Geometry check sheet. Reference: the model listing, model coordinates, mm. Round coordinates to 2 decimals unless told otherwise and drop trailing zeros. Loops run counter-clockwise (first coordinate to the right, second up) from the corner with the lowest first, then second, coordinate; pieces in that order, holes last. Notation, with made-up numbers: (-2, 78.25) -> (50, 78.25) arc R30 cw to (50, 107.25) -> close; hole circle Ø8 at (5.5, -11.75). An arc over 180 degrees is marked (long way). Use one line per item in the form item = value.
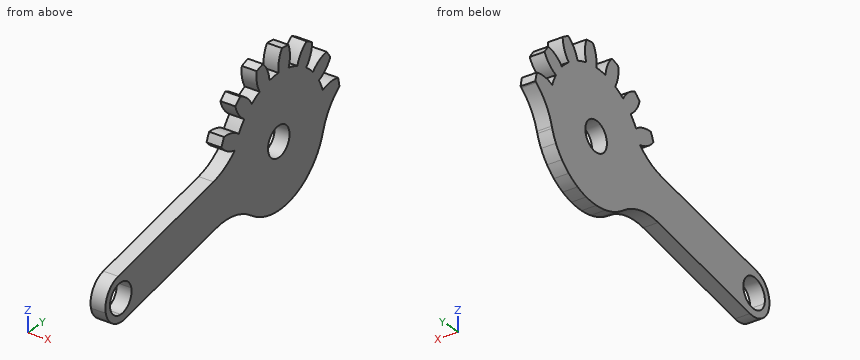
from build123d import *

# Parameters (mm, degrees)
SKETCH1_R           = 1.5
BOSS_EXTRUDE1_DEPTH = 2
SKETCH3_OUTSIDE_W   = 31.914
SKETCH3_OUTSIDE_H   = 31.796
SKETCH3_OUTSIDE_R   = 11.40725
CUT_EXTRUDE1_DEPTH  = 17.630863493
SKETCH4_R           = 2
CUT_EXTRUDE2_DEPTH  = 17.245136509
BOSS_EXTRUDE3_DEPTH = 2
CUT_EXTRUDE3_DEPTH  = 35.211805454
FILLET1_R           = 8


with BuildPart() as part:
    # Sketch1 → Boss-Extrude1 (new body)
    with BuildSketch(Plane(origin=(-1.354941904, 0, 0), x_dir=(0, 0, -1), z_dir=(1, 0, 0))):
        with BuildLine():
            ThreePointArc((-11.66138775, 0.780827758), (-10.210393031, 0.057188521), (-8.592596732, -0.051322118))
            ThreePointArc((-8.592596732, -0.051322118), (-8.545678016, -0.898186953), (-8.415498346, -1.736300708))
            ThreePointArc((-8.415498346, -1.736300708), (-9.975381284, -2.178798893), (-11.24421523, -3.188303642))
            ThreePointArc((-11.24421523, -3.188303642), (-11.115473034, -3.611636122), (-10.97079907, -4.029792056))
            ThreePointArc((-10.97079907, -4.029792056), (-9.350918841, -4.100696673), (-7.828853128, -3.541809038))
            ThreePointArc((-7.828853128, -3.541809038), (-7.441539788, -4.296375), (-6.981723166, -5.009081172))
            ThreePointArc((-6.981723166, -5.009081172), (-8.226766912, -6.047784929), (-8.975301827, -7.486094667))
            ThreePointArc((-8.975301827, -7.486094667), (-8.685505148, -7.820463962), (-8.383259564, -8.143624213))
            ThreePointArc((-8.383259564, -8.143624213), (-6.874585833, -7.549534157), (-5.711429695, -6.419884999))
            ThreePointArc((-5.711429695, -6.419884999), (-5.050691727, -6.951680778), (-4.340744624, -7.415745996))
            ThreePointArc((-4.340744624, -7.415745996), (-5.055669804, -8.871054007), (-5.154477201, -10.489471914))
            ThreePointArc((-5.154477201, -10.489471914), (-4.753734516, -10.677062536), (-4.34617832, -10.849349762))
            ThreePointArc((-4.34617832, -10.849349762), (-3.209574481, -9.692988601), (-2.606448181, -8.187904521))
            ThreePointArc((-2.606448181, -8.187904521), (-1.786533181, -8.404977796), (-0.949211902, -8.540160966))
            ThreePointArc((-0.949211902, -8.540160966), (-1.010401457, -10.160437258), (-0.442396639, -11.679124174))
            ThreePointArc((-0.442396639, -11.679124174), (0, -11.6875), (0.442396639, -11.679124174))
            ThreePointArc((0.442396639, -11.679124174), (1.010401457, -10.160437258), (0.949211902, -8.540160966))
            ThreePointArc((0.949211902, -8.540160966), (1.786533181, -8.404977796), (2.606448181, -8.187904521))
            ThreePointArc((2.606448181, -8.187904521), (3.209574481, -9.692988601), (4.34617832, -10.849349762))
            ThreePointArc((4.34617832, -10.849349762), (4.753734516, -10.677062536), (5.154477201, -10.489471914))
            ThreePointArc((5.154477201, -10.489471914), (5.055669804, -8.871054007), (4.340744624, -7.415745996))
            ThreePointArc((4.340744624, -7.415745996), (5.050691727, -6.951680778), (5.711429695, -6.419884999))
            ThreePointArc((5.711429695, -6.419884999), (6.874585833, -7.549534157), (8.383259564, -8.143624213))
            ThreePointArc((8.383259564, -8.143624213), (8.685505148, -7.820463962), (8.975301827, -7.486094667))
            ThreePointArc((8.975301827, -7.486094667), (8.226766912, -6.047784929), (6.981723166, -5.009081172))
            ThreePointArc((6.981723166, -5.009081172), (7.441539788, -4.296375), (7.828853128, -3.541809038))
            ThreePointArc((7.828853128, -3.541809038), (9.350918841, -4.100696673), (10.97079907, -4.029792056))
            ThreePointArc((10.97079907, -4.029792056), (11.115473034, -3.611636122), (11.24421523, -3.188303642))
            ThreePointArc((11.24421523, -3.188303642), (9.975381284, -2.178798893), (8.415498346, -1.736300708))
            ThreePointArc((8.415498346, -1.736300708), (8.545678016, -0.898186953), (8.592596732, -0.051322118))
            ThreePointArc((8.592596732, -0.051322118), (10.210393031, 0.057188521), (11.66138775, 0.780827758))
            ThreePointArc((11.66138775, 0.780827758), (11.623474652, 1.221676414), (11.568901669, 1.660774047))
            ThreePointArc((11.568901669, 1.660774047), (9.999161608, 2.066921265), (8.394157409, 1.836701922))
            ThreePointArc((8.394157409, 1.836701922), (8.17219088, 2.655305778), (7.8706023, 3.448038862))
            ThreePointArc((7.8706023, 3.448038862), (9.304397507, 4.205185299), (10.335616548, 5.456435359))
            ThreePointArc((10.335616548, 5.456435359), (10.121671907, 5.84375), (9.893219909, 6.222688815))
            ThreePointArc((9.893219909, 6.222688815), (8.29399605, 5.955251959), (6.921390398, 5.092122104))
            ThreePointArc((6.921390398, 5.092122104), (6.385657699, 5.749672018), (5.787709228, 6.351202599))
            ThreePointArc((5.787709228, 6.351202599), (6.789587127, 7.626067336), (7.222723349, 9.188575716))
            ThreePointArc((7.222723349, 9.188575716), (6.869740136, 9.455386122), (6.506910549, 9.708644156))
            ThreePointArc((6.506910549, 9.708644156), (5.154723227, 8.813865487), (4.251852108, 7.467068114))
            ThreePointArc((4.251852108, 7.467068114), (3.49498629, 7.849867731), (2.704068651, 8.156185707))
            ThreePointArc((2.704068651, 8.156185707), (3.100795451, 9.728333051), (2.860955666, 11.331927856))
            ThreePointArc((2.860955666, 11.331927856), (2.429967886, 11.432100084), (1.995497243, 11.515886722))
            ThreePointArc((1.995497243, 11.515886722), (1.124151929, 10.148481601), (0.847129962, 8.55089021))
            ThreePointArc((0.847129962, 8.55089021), (0, 8.59275), (-0.847129962, 8.55089021))
            ThreePointArc((-0.847129962, 8.55089021), (-1.124151929, 10.148481601), (-1.995497243, 11.515886722))
            ThreePointArc((-1.995497243, 11.515886722), (-2.429967886, 11.432100084), (-2.860955666, 11.331927856))
            ThreePointArc((-2.860955666, 11.331927856), (-3.100795451, 9.728333051), (-2.704068651, 8.156185707))
            ThreePointArc((-2.704068651, 8.156185707), (-3.49498629, 7.849867731), (-4.251852108, 7.467068114))
            ThreePointArc((-4.251852108, 7.467068114), (-5.154723227, 8.813865487), (-6.506910549, 9.708644156))
            ThreePointArc((-6.506910549, 9.708644156), (-6.869740136, 9.455386122), (-7.222723349, 9.188575716))
            ThreePointArc((-7.222723349, 9.188575716), (-6.789587127, 7.626067336), (-5.787709228, 6.351202599))
            ThreePointArc((-5.787709228, 6.351202599), (-6.385657699, 5.749672018), (-6.921390398, 5.092122104))
            ThreePointArc((-6.921390398, 5.092122104), (-8.29399605, 5.955251959), (-9.893219909, 6.222688815))
            ThreePointArc((-9.893219909, 6.222688815), (-10.121671907, 5.84375), (-10.335616548, 5.456435359))
            ThreePointArc((-10.335616548, 5.456435359), (-9.304397507, 4.205185299), (-7.8706023, 3.448038862))
            ThreePointArc((-7.8706023, 3.448038862), (-8.17219088, 2.655305778), (-8.394157409, 1.836701922))
            ThreePointArc((-8.394157409, 1.836701922), (-9.999161608, 2.066921265), (-11.568901669, 1.660774047))
            ThreePointArc((-11.568901669, 1.660774047), (-11.623474652, 1.221676414), (-11.66138775, 0.780827758))
        make_face()
        with Locations(Location((0, 0, 0), (0, 0, 180))):
            Circle(SKETCH1_R, mode=Mode.SUBTRACT)
    extrude(amount=-BOSS_EXTRUDE1_DEPTH)

    # Sketch3 outside → Cut-Extrude1 (cut, through all)
    with BuildSketch(Plane(origin=(-1.354941904, 0, 0), x_dir=(0, 0, -1), z_dir=(1, 0, 0))):
        with Locations((0, -0.086)):
            Rectangle(SKETCH3_OUTSIDE_W, SKETCH3_OUTSIDE_H)
        Circle(SKETCH3_OUTSIDE_R, mode=Mode.SUBTRACT)
    extrude(amount=-CUT_EXTRUDE1_DEPTH, mode=Mode.SUBTRACT)

    # Sketch4 → Cut-Extrude2 (cut, through all)
    with BuildSketch(Plane.ZY.offset(3.354941904)):
        Circle(SKETCH4_R)
    extrude(amount=-CUT_EXTRUDE2_DEPTH, mode=Mode.SUBTRACT)

    # Sketch5 → Boss-Extrude3 (add)
    with BuildSketch(Plane(origin=(-1.354941904, 0, 0), x_dir=(0, 0, -1), z_dir=(1, 0, 0))):
        with BuildLine():
            Line((5.821527343, -27.388132821), (0.895701941, -4.213946322))
            Line((0.895701941, -4.213946322), (-2.171319843, -4.213946322))
            Line((-2.171319843, -4.213946322), (3.27164281, -29.821072303))
            ThreePointArc((3.27164281, -29.821072303), (4.572168507, -31.713348935), (6.829820684, -32.131780033))
            Line((6.829820684, -32.131780033), (6.653174106, -31.300723223))
            ThreePointArc((6.653174106, -31.300723223), (4.281055523, -29.760251404), (5.821527343, -27.388132821))
        make_face()
        with BuildLine():
            Line((3.962723726, -4.213946322), (0.895701941, -4.213946322))
            Line((0.895701941, -4.213946322), (5.821527343, -27.388132821))
            ThreePointArc((5.821527343, -27.388132821), (7.495991507, -27.790136099), (8.237350725, -29.344428022))
            ThreePointArc((8.237350725, -29.344428022), (7.791642647, -30.603068804), (6.653174106, -31.300723223))
            Line((6.653174106, -31.300723223), (6.829820684, -32.131780033))
            ThreePointArc((6.829820684, -32.131780033), (8.722097316, -30.831254336), (9.140528414, -28.573602159))
            Line((9.140528414, -28.573602159), (3.962723726, -4.213946322))
        make_face()
    extrude(amount=-BOSS_EXTRUDE3_DEPTH)

    # Sketch6 → Cut-Extrude3 (cut, through all)
    with BuildSketch(Plane(origin=(-1.354941904, 0, 0), x_dir=(0, 0, -1), z_dir=(1, 0, 0))):
        with BuildLine():
            ThreePointArc((4.60855611, -7.252348802), (8.250847615, 2.39976378), (0, 8.59275))
            Line((0, 8.59275), (0, 11.449359201))
            ThreePointArc((0, 11.449359201), (11.128561829, 2.691270657), (5.231728933, -10.184146429))
            Line((5.231728933, -10.184146429), (4.60855611, -7.252348802))
        make_face()
        with BuildLine():
            ThreePointArc((-1.878840334, -8.384826269), (-1.570637651, -8.447984963), (-1.260329494, -8.499818947))
            Line((-1.260329494, -8.499818947), (-0.637156671, -11.431616574))
            ThreePointArc((-0.637156671, -11.431616574), (-1.575646482, -11.340421698), (-2.503449753, -11.172312449))
            Line((-2.503449753, -11.172312449), (-1.878840334, -8.384826269))
        make_face()
    extrude(amount=-CUT_EXTRUDE3_DEPTH, mode=Mode.SUBTRACT)

    # Fillet1
    # the kernel refuses this fillet: 8 mm, written as the material it adds along each edge
    with BuildSketch(Plane(origin=(-3.354941904, -8.499818947, 1.260329494), x_dir=(0, -0.978147600733804, -0.20791169081776692), z_dir=(1, 0, 0))) as fillet1_piece_1:
        with BuildLine():
            CenterArc((3.711828979, -8), FILLET1_R, 90, 32.486450305)
            Line((-0.58497216, -1.251852108), (-0.670908182, -1.11688915))
            ThreePointArc((-0.670908182, -1.11688915), (-0.412236702, -0.569968342), (-0.149931796, 0.055861046))
            Line((-0.149931796, 0.055861046), (0, 0.16))
            Line((0, 0.16), (3.711828979, 0.16))
            Line((3.711828979, 0.16), (3.711828979, 0))
        make_face()
    extrude(amount=2)
    with BuildSketch(Plane(origin=(-3.354941904, -7.252348802, -4.60855611), x_dir=(0, 0.6817347093363165, -0.7315994710810882), z_dir=(1, 0, 0))) as fillet1_piece_2:
        with BuildLine():
            CenterArc((4.609202788, -7.864888151), FILLET1_R, 100.545143381, 48.475508098)
            Line((-2.24962028, -3.747055453), (-2.386796741, -3.664698799))
            Line((-2.386796741, -3.664698799), (-0.137176461, 0.082356654))
            Line((-0.137176461, 0.082356654), (0.029281628, 0.157297763))
            ThreePointArc((0.029281628, 0.157297763), (1.57256069, 0.014877208), (3.115839752, 0.157297763))
            Line((3.115839752, 0.157297763), (3.14512138, 0))
        make_face()
    extrude(amount=2)
    with BuildSketch(Plane(origin=(-1.354941904, 8.55089021, 0.847129962), x_dir=(0, 0.9533192219499187, 0.3019643373989743), z_dir=(-1, 0, 0))) as fillet1_piece_3:
        with BuildLine():
            CenterArc((5.310026661, 7.560828727), FILLET1_R, 214.236741242, 36.690361487)
            Line((-1.30373306, 3.059919669), (-1.436008254, 2.969901488))
            ThreePointArc((-1.436008254, 2.969901488), (-0.64959553, 1.530927434), (-0.156551158, -0.03304141))
            Line((-0.156551158, -0.03304141), (0.052283339, -0.151216575))
            ThreePointArc((0.052283339, -0.151216575), (1.347929845, 0.066447687), (2.64357635, -0.151216575))
            Line((2.64357635, -0.151216575), (2.69585969, 0))
        make_face()
    extrude(amount=2)


solid = part.part
1. Section check A-A (z = 0). Record the boundary of the cut face in (x, y).
Return value:
outline = (-3.35, -14.43) -> (-1.35, -14.43) -> (-1.35, -2) -> (-3.35, -2) -> close; (-3.35, 2) -> (-1.35, 2) -> (-1.35, 9.46) -> (-3.35, 9.46) -> close
2. Material ranges on line 1 along Z through (x, y) = (-2.05, -9); line 2 along Z through (x, y) = (-2.65, 9); line 3 along Y through (x, z) = (-1.6, -4.5), recorded low to high.
Return value:
line_1 = -5.39 to 1.91, 2.85 to 5.09
line_2 = -0.7 to 3, 5.35 to 7.01
line_3 = -31.66 to -30.34, -28.35 to 7.32
3. Section check B-B (x = -2.45). Count the separate pieces of the cut face and the enclosed holes in it, then the cut area to 3 significant figures.
Return value:
separate_pieces = 1
enclosed_holes = 2
area = 393 mm2
4. Gauge pin test, flat end, axial feed: pin 1 (10 mm diameter, centred on y = -25.5, z = -1.5, fed in from +X). Record the tip position at first contact, or that the pin passes through.
Return value:
pin_1 = -1.35
5. Section check D-D (y = -13). Record the boundary of the cut face in (x, z), then the cut area to 3 significant figures.
Return value:
outline = (-3.35, -5.83) -> (-1.35, -5.83) -> (-1.35, 0.3) -> (-3.35, 0.3) -> close
area = 12.3 mm2
6. Section check C-C (y = 4.5). Record the boundary of the cut face in (x, z), then the cut area to 3 significant figures.
Return value:
outline = (-3.35, -7.32) -> (-1.35, -7.32) -> (-1.35, 9.63) -> (-3.35, 9.63) -> close
area = 33.9 mm2
